Here's how the part is built. I have some questions about the finished solid (model axes, mm). A direction names the side the tool comes from. Coordinates: 2 decimals unless noted, no trailing zeros. Loops run counter-clockwise (first coordinate to the right, second up) from the corner with the lowest first, then second, coordinate; pieces in that order, holes last. Notation, with made-up numbers: M 76.25,2 L 130.25,2 A21 cw 130.25,31 Z; hole C 55,52.5 d1. An arc over 180 degrees is marked long. Use one line per item in the form item = value. Start each with the question number.
(1) Thinking about a two-plate mould opening in X: for faces 1 (the flat face through (52, 1, -35.75)), 2 (the flat face through (52, 36, 36)), 3 (the flat face through (-55, 17, 1)), which applies, +X half, -X half, draft (parallel to the pull), parting line (faces both ways), or undercut?
(2) On a 3-axis mill with a long thin cutter (end or side, diameter ignored), from which of +Z, -Z, +X, -X, +Y, -Y can I reach the whole of each face in a straight line? I mean faces 4 (the flat face through (-51, 36, -37)), 5 (the flat face through (-1, 0, -1)), 6 (the flat face through (21.631, 3, 30)), 7 (the flat face through (-54.25, 1, -38)), 8 (the flat face through (-1, 24, -35)). Say none if no direction works.
(3) Imagine slicing it at B-B, the plane x = 24. Please give me the cut outline in (y, z), and give its area (3 significant figures).
(4) Imagine slicing it at C-C, the plane x = 10. Please give me the cut outline in (y, z).
(5) Imagine slicing it at A-A, the plane z = 29. Please give me the cut outline in (x, y), and give its area (3 significant figures).
(6) Will these pins go through, and if not, where does the flat tip stop? P1, Ø2.5, axis at x = 52, y = 36, coming from the -Z side; P2, Ø0.9, axis at x = -52.5, y = 36.5, coming from the +Z side; P3, Ø1, axis at x = -52.5, z = -37, coming from the -Y side; P4, Ø10, axis at x = 33.5, z = 4, coming from the +Y side.
(7) Imagine slicing it at D-D, the plane y = 28. Please give me the cut outline in (x, z).
(8) Please list where these lines run through material, in increasing order: L1, parallel to Z at x = 16, y = 33.5; L2, parallel to X at y = 30, z = -27.5; L3, parallel to Z at x = -12.5, y = 3.
```python
from build123d import *

# Parameters (mm, degrees)
SKETCH_1_W          = 110
SKETCH_1_H          = 80
EXTRUDE_1_DEPTH     = 5
SKETCH_3_W          = 3.5
SKETCH_3_H          = 3.5
CUT_EXTRUDE_1_DEPTH = 3
SKETCH_4_W          = 58
SKETCH_4_H          = 5
CUT_EXTRUDE_2_DEPTH = 5
SKETCH_5_W          = 110
SKETCH_5_H          = 80
EXTRUDE_2_DEPTH     = 30
SKETCH_7_W          = 100
SKETCH_7_H          = 70
CUT_EXTRUDE_3_DEPTH = 30
SKETCH_8_W          = 3
SKETCH_8_H          = 3
EXTRUDE_3_DEPTH     = 3
SKETCH_9_W          = 70
SKETCH_9_H          = 12
CUT_EXTRUDE_4_DEPTH = 10


with BuildPart() as part:
    # 스케치1 → 보스-돌출1 (new body)
    with BuildSketch(Plane(origin=(0, 0, 0), x_dir=(1, 0, 0), z_dir=(0, 1, 0))):
        Rectangle(SKETCH_1_W, SKETCH_1_H)
    extrude(amount=EXTRUDE_1_DEPTH)

    # 스케치3 → 컷-돌출1 (cut)
    with BuildSketch(Plane.XZ):
        with Locations((-52.5, 37.5)):
            Rectangle(SKETCH_3_W, SKETCH_3_H)
        with Locations((52.5, 37.5)):
            Rectangle(SKETCH_3_W, SKETCH_3_H)
        with Locations((-52.5, -37.5)):
            Rectangle(SKETCH_3_W, SKETCH_3_H)
        with Locations((52.5, -37.5)):
            Rectangle(SKETCH_3_W, SKETCH_3_H)
    extrude(amount=-CUT_EXTRUDE_1_DEPTH, mode=Mode.SUBTRACT)

    # 스케치4 → 컷-돌출2 (cut)
    with BuildSketch(Plane(origin=(0, 5, 0), x_dir=(1, 0, 0), z_dir=(0, 1, 0))):
        with Locations((-7.368635656, -29.764338216)):
            Rectangle(SKETCH_4_W, SKETCH_4_H)
    extrude(amount=-CUT_EXTRUDE_2_DEPTH, mode=Mode.SUBTRACT)

    # 스케치5 → 보스-돌출2 (add)
    with BuildSketch(Plane(origin=(0, 5, 0), x_dir=(1, 0, 0), z_dir=(0, 1, 0))):
        Rectangle(SKETCH_5_W, SKETCH_5_H)
    extrude(amount=EXTRUDE_2_DEPTH)

    # 스케치7 → 컷-돌출3 (cut)
    with BuildSketch(Plane(origin=(0, 35, 0), x_dir=(1, 0, 0), z_dir=(0, 1, 0))):
        Rectangle(SKETCH_7_W, SKETCH_7_H)
    extrude(amount=-CUT_EXTRUDE_3_DEPTH, mode=Mode.SUBTRACT)

    # 스케치8 → 보스-돌출3 (add)
    with BuildSketch(Plane(origin=(0, 35, 0), x_dir=(1, 0, 0), z_dir=(0, 1, 0))):
        with Locations((-52.5, 37.5)):
            Rectangle(SKETCH_8_W, SKETCH_8_H)
        with Locations((-52.5, -37.5)):
            Rectangle(SKETCH_8_W, SKETCH_8_H)
        with Locations((52.5, -37.5)):
            Rectangle(SKETCH_8_W, SKETCH_8_H)
        with Locations((52.5, 37.5)):
            Rectangle(SKETCH_8_W, SKETCH_8_H)
    extrude(amount=EXTRUDE_3_DEPTH)

    # 스케치9 → 컷-돌출4 (cut)
    with BuildSketch(Plane(origin=(0, 0, -40), x_dir=(-1, 0, 0), z_dir=(0, 0, -1))):
        with Locations((2.129578344, 16.097594135)):
            Rectangle(SKETCH_9_W, SKETCH_9_H)
    extrude(amount=-CUT_EXTRUDE_4_DEPTH, mode=Mode.SUBTRACT)


solid = part.part
```
Answer:
q1.face_1 = undercut
q1.face_2 = draft
q1.face_3 = -X half
q2.face_4 = +Z, -Z, +Y
q2.face_5 = +Z, -Z, +X, -X, -Y
q2.face_6 = +Y, -Y
q2.face_7 = -Y
q2.face_8 = +Y
q3.outline = M 0,-40 L 10.1,-40 L 10.1,-35 L 5,-35 L 5,35 L 35,35 L 35,40 L 0,40 Z; M 22.1,-40 L 35,-40 L 35,-35 L 22.1,-35 Z
q3.area = 640 mm²
q4.outline = M 0,-40 L 10.1,-40 L 10.1,-35 L 5,-35 L 5,27.26 L 0,27.26 Z; M 0,32.26 L 5,32.26 L 5,35 L 35,35 L 35,40 L 0,40 Z; M 22.1,-40 L 35,-40 L 35,-35 L 22.1,-35 Z
q5.outline = M -55,0 L -36.37,0 L -36.37,5 L -50,5 L -50,35 L -55,35 Z; M 21.63,0 L 55,0 L 55,35 L 50,35 L 50,5 L 21.63,5 Z
q5.area = 560 mm²
q6.P1 = -40
q6.P2 = 39
q6.P3 = 3
q6.P4 = 5
q7.outline = M -55,-40 L 55,-40 L 55,40 L -55,40 Z; hole M -50,-35 L 50,-35 L 50,35 L -50,35 Z
q8.L1 = -40 to -35, 35 to 40
q8.L2 = -55 to -50, 50 to 55
q8.L3 = -40 to 27.26, 32.26 to 40
